```python
from build123d import *

# Parameters (mm, degrees)
SKETCH_1_W      = 16
SKETCH_1_H      = 80
SKETCH_1_R      = 2.25
EXTRUDE_1_DEPTH = 80
EXTRUDE_2_DEPTH = 16


with BuildPart() as part:
    # 草图1 → 凸台-拉伸1 (new body)
    with BuildSketch(Plane.XY):
        Rectangle(SKETCH_1_W, SKETCH_1_H)
        with Locations((0, 32)):
            Circle(SKETCH_1_R, mode=Mode.SUBTRACT)
        Circle(SKETCH_1_R, mode=Mode.SUBTRACT)
        with Locations((0, -32)):
            Circle(SKETCH_1_R, mode=Mode.SUBTRACT)
    extrude(amount=EXTRUDE_1_DEPTH)

    # 草图2 → 凸台-拉伸2 (add)
    with BuildSketch(Plane(origin=(8, 0, 0), x_dir=(0, 0, -1), z_dir=(1, 0, 0))):
        Polygon((-80, -40), (-100.37264984, 3.68928857), (-158.198670132, 127.697589274), (-83.944773743, 127.697589274), (-43.050716263, 40), align=None)
    extrude(amount=-EXTRUDE_2_DEPTH)


solid = part.part
```
Source: CAD feature listing. Evaluate the final solid. Frame: model axes, mm. A direction names the side the tool comes from. Coordinates: 2 decimals unless noted, no trailing zeros. Loops run counter-clockwise (first coordinate to the right, second up) from the corner with the lowest first, then second, coordinate; pieces in that order, holes last. Notation, with made-up numbers: M 6,19 L 17,19 A22 cw 17,54 Z; hole C -8.75,1 d3. An arc over 180 degrees is marked long. Use CSV: the item, a comma, the result in double quotes.
(1) Cut plane A-A on z = 22.5. Return loops of the section in (x, y), and give its area (3 significant figures).
Answers follow:
outline,"M -8,-40 L 8,-40 L 8,40 L -8,40 Z; hole C 0,-32 d4.5; hole C 0,0 d4.5; hole C 0,32 d4.5"
area,"1,230 mm²"
(2) Draft query along X for faces 1 (the face through (0.03, 0.03, 61.51)), 2 (the face through (-8, 45, 78)), 3 (the face through (0.03, -31.97, 76.29)), 4 (the face through (0, 40, 21)). Return one class per face: pulls with the +X half, pulls with the -X half, needs draft (parallel to the pull), parting line crosses it, or undercut.
Answers follow:
face 1,"undercut"
face 2,"pulls with the -X half"
face 3,"undercut"
face 4,"needs draft"
(3) Line query: line 1 (Y direction, x = 0, z = 31.5); line 2 (X direction, y = 32, z = 12); line 3 (Y direction, x = 0, z = 46). Output: solid intervals per line, ascending. Write a range as [from, to].
Answers follow:
line 1,"[-40, -34.25], [-29.75, -2.25], [2.25, 29.75], [34.25, 40]"
line 2,"[-8, -2.25], [2.25, 8]"
line 3,"[-40, -34.25], [-29.75, -2.25], [2.25, 29.75], [33.61, 46.32]"
(4) Reachability of faces 5 (the face through (8, 45, 78)), 6 (the face through (-0.29, 34.23, 23.57)) from +Z, -Z, +X, -X, +Y, -Y: full face, straight path, thin tool, end or side. Return the list, or none.
Answers follow:
face 5,"+Z, -Z, +X, +Y, -Y"
face 6,"-Z"
(5) Cut plane B-B on x = 6. Return loops of the section in (y, z).
Answers follow:
outline,"M -40,0 L 40,0 L 40,43.05 L 127.7,83.94 L 127.7,158.2 L -40,80 Z"
(6) Cut plane C-C on y = 0. Return loops of the section in (x, z).
Answers follow:
outline,"M -8,0 L -2.25,0 L -2.25,61.53 L 2.25,61.53 L 2.25,0 L 8,0 L 8,98.65 L -8,98.65 Z"
(7) Contact query for flat-ended pins moving along their axis: pin 1 (4 mm diameter, centred on x = 0, y = -32, fed in from -Z); pin 2 (3.5 mm diameter, centred on x = 0, y = 32, fed in from -Z); pin 3 (3.5 mm diameter, centred on x = 0, y = 0, fed in from +Z). Output: stop coordinate, or through.
Answers follow:
pin 1,"z = 75.38"
pin 2,"z = 45.94"
pin 3,"z = 99.47"
(8) Cut plane D-D on z = 96. Return loops of the section in (x, y).
Answers follow:
outline,"M -8,-5.69 L 8,-5.69 L 8,127.7 L -8,127.7 Z"
